from build123d import *

# Parameters (mm, degrees)
F0_R     = 5
F1_DEPTH = 10
F2_T     = -1.1
F4_DEPTH = 8.9
F5_R     = 0.5


with BuildPart() as f1:
    # F0 (on Top) → F1 (new body)
    with BuildSketch(Plane.XY):
        Circle(F0_R)
    extrude(amount=F1_DEPTH)

    # F2
    f2_openings = [f1.faces().sort_by_distance(p)[0] for p in [
        (0, 0, 10),
    ]]
    offset(amount=F2_T, openings=f2_openings)

    # F3 (on face) → F4 (join, through all)
    with BuildSketch(Plane.XY.offset(1.1)):
        with BuildLine():
            Line((-0.55, 0.55), (-3.861023, 0.55))
            ThreePointArc((-3.861023, 0.55), (-3.9, 0), (-3.861023, -0.55))
            Line((-3.861023, -0.55), (-0.55, -0.55))
            Line((-0.55, -0.55), (-0.55, -3.861023))
            ThreePointArc((-0.55, -3.861023), (0, -3.9), (0.55, -3.861023))
            Line((0.55, -3.861023), (0.55, -0.55))
            Line((0.55, -0.55), (3.861023, -0.55))
            ThreePointArc((3.861023, -0.55), (3.9, 0), (3.861023, 0.55))
            Line((3.861023, 0.55), (0.55, 0.55))
            Line((0.55, 0.55), (0.55, 3.861023))
            ThreePointArc((0.55, 3.861023), (0, 3.9), (-0.55, 3.861023))
            Line((-0.55, 3.861023), (-0.55, 0.55))
        make_face()
    extrude(amount=F4_DEPTH)

    # F5
    f5_edges = [f1.edges().sort_by_distance(p)[0] for p in [
        (-5, 0, 10),
        (-5, 0, 0),
    ]]
    fillet(f5_edges, radius=F5_R)


solid = f1.part
Source: CAD feature listing. Evaluate the final solid. Frame: model axes, mm. A direction names the side the tool comes from. Round coordinates to 2 decimals unless told otherwise and drop trailing zeros. Loops run counter-clockwise (first coordinate to the right, second up) from the corner with the lowest first, then second, coordinate; pieces in that order, holes last.
Q1. Access query for faces 5 (the face through (0, 0, 0)), 6 (the face through (2, -0.55, 5)). Directions: +Z, -Z, +X, -X, +Y, -Y. A direction counts if a zero-diameter tool reaches every point of the face in a straight line with its end or side. Return the directions, or none.
Q2. Ray query, line 1 (Y direction, x = 2, z = 9.75); line 2 (X direction, y = 1, z = 9.75); line 3 (Y direction, x = 1.75, z = 1.25). Return the intervals inside material, ascending.
Q3. Mould query, pull axis Y, two halves, no side actions, for faces 1 (the face through (-2, 2, 1.1)), 2 (the face through (-2.733, 2.782, 5.488)), 3 (the face through (-1.08, -4.88, 4.94)), 4 (the face through (0, 0, 10)). Classes: pulls with the +Y half, pulls with the -Y half, needs draft (parallel to the pull), parting line crosses it, or undercut.
Q4. Section A-A, the plane z = 5.5. Return loops of the section in (x, y), plus the area to 3 significant figures.
Q5. First-contact query: P1, Ø1.7, axis at x = 3, z = 4.5, coming from the +Y side; P2, Ø4, axis at y = -3.5, z = 5.5, coming from the +X side; P3, Ø2.5, axis at y = -2.5, z = 4.5, coming from the -X side. Flat tips, straight axial feed; report the tip coordinate or a pass-through.
Solutions:
1. face 5: -Z, +X, -X, +Y, -Y
1. face 6: +Z
2. line 1: y = -4.51 to -3.35, -0.55 to 0.55, 3.35 to 4.51
2. line 2: x = -4.83 to -3.77, -0.55 to 0.55, 3.77 to 4.83
2. line 3: y = -4.68 to -3.49, -0.55 to 0.55, 3.49 to 4.68
3. face 1: undercut
3. face 2: undercut
3. face 3: parting line crosses it
3. face 4: needs draft
4. outline: circle Ø10 at (0, 0); hole (-3.86, -0.55) arc R3.9 ccw to (-0.55, -3.86) - (-0.55, -0.55) - close; hole (-3.86, 0.55) - (-0.55, 0.55) - (-0.55, 3.86) arc R3.9 ccw to start; hole (0.55, -3.86) arc R3.9 ccw to (3.86, -0.55) - (0.55, -0.55) - close; hole (0.55, 0.55) - (3.86, 0.55) arc R3.9 ccw to (0.55, 3.86) - close
4. area: 46.6 mm2
5. P1: stops at y = 4.51
5. P2: stops at x = 4.77
5. P3: stops at x = -4.84
